Answer from the drawing. Dimensions are ordinates in mm from the lowest x, y and z of the part. A direction names the side the tool comes from. Coordinates: 2 decimals unless noted, no trailing zeros. Write each loop counter-clockwise with the first axis right and the second up, starting at its lowest first coordinate (ties: lowest second). Pieces come first, ordered by that corner, then holes. Notation, with made-up numbers: (-40, -30.5) - (-16, -30.5) arc R20 cw to (-16, 5.5) - close; hole circle Ø3 at (-31, 25.5). An arc over 180 degrees is marked (long way). Return JSON: item names as keys, results as strings.
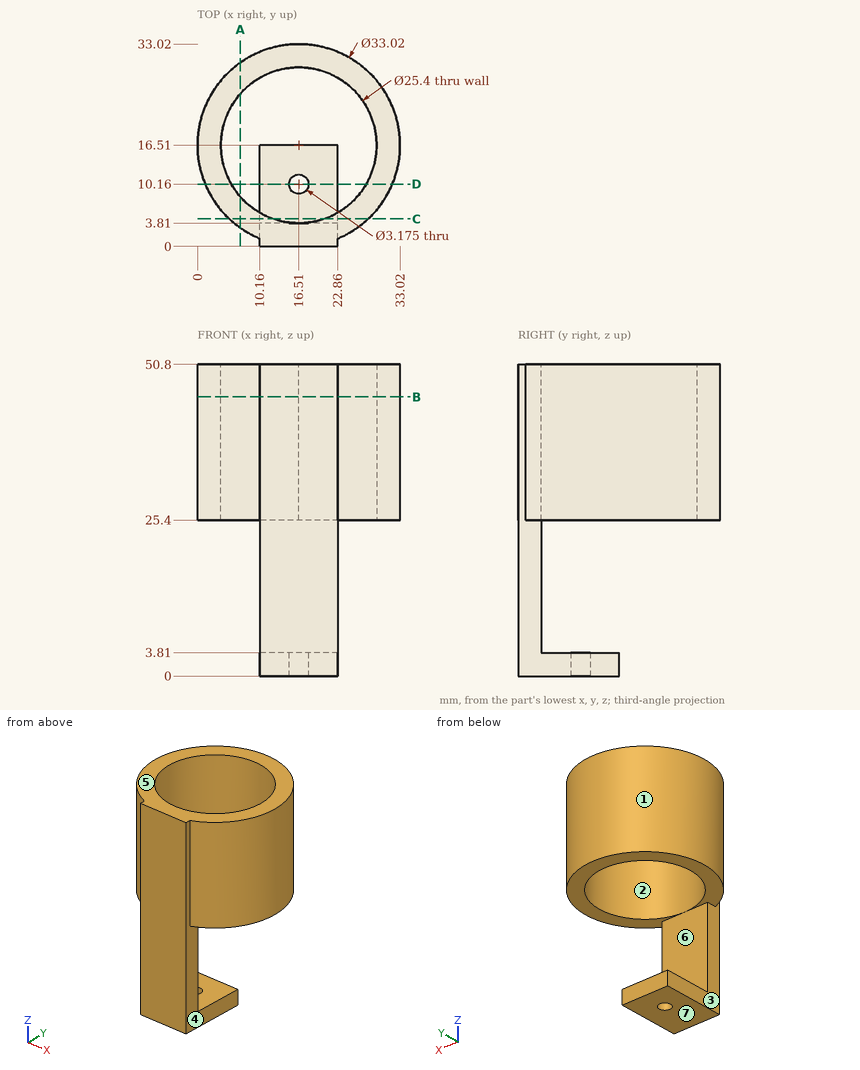
(1) Which of the six approach directions +Z, -Z, +X, -X, +Y, -Y give full straight-line access (tool end or side, diameter ignored) to the marked faces 1, 2 and 3?
Answer:
{"face 1": "+Z, -Z", "face 2": "+Z", "face 3": "-Z, -X, -Y"}
(2) A cutting plane is placed at C-C (y = 4.5). Determine the outline of the cut face in (x, z), and give its area (3 significant figures).
Answer:
{"outline": "(5.18, 25.4) - (12.38, 25.4) - (12.38, 50.8) - (5.18, 50.8) - close; (10.16, 0) - (22.86, 0) - (22.86, 3.81) - (10.16, 3.81) - close; (20.64, 25.4) - (27.84, 25.4) - (27.84, 50.8) - (20.64, 50.8) - close", "area": "414 mm²"}
(3) A cutting plane is placed at D-D (y = 10.16). Determine the outline of the cut face in (x, z).
Answer:
{"outline": "(1.27, 25.4) - (5.51, 25.4) - (5.51, 50.8) - (1.27, 50.8) - close; (10.16, 0) - (14.92, 0) - (14.92, 3.81) - (10.16, 3.81) - close; (18.1, 0) - (22.86, 0) - (22.86, 3.81) - (18.1, 3.81) - close; (27.51, 25.4) - (31.75, 25.4) - (31.75, 50.8) - (27.51, 50.8) - close"}
(4) Flat-ended cylindrical pins translate along their axes: P1, Ø8, axis at y = 8.5, z = 39.5, coming from the -X side; P2, Ø1.9, axis at x = 18.5, z = 1.5, coming from the +Y side; P3, Ø9.5, axis at x = 12.5, y = 24.5, coming from the -Z side. Find the tip coordinate at first contact, or state that the pin passes through.
Answer:
{"P1": "x = 0.49", "P2": "y = 16.51", "P3": "z = 25.4"}
(5) A cutting plane is placed at A-A (x = 7). Determine the outline of the cut face in (y, z), and give its area (3 significant figures).
Answer:
{"outline": "(3.01, 25.4) - (8.09, 25.4) - (8.09, 50.8) - (3.01, 50.8) - close; (24.93, 25.4) - (30.01, 25.4) - (30.01, 50.8) - (24.93, 50.8) - close", "area": "258 mm²"}
(6) Straight lines are drawn through the part: line 1 (X direction, y = 16, z = 42); line 2 (X direction, y = 10, z = 1); line 3 (Z direction, x = 22, y = 28). For each, find the intervals that lie inside material, in ascending order. Write a range as from..to.
Answer:
{"line 1": "0.01..3.82, 29.2..33.01", "line 2": "10.16..14.93, 18.09..22.86", "line 3": "25.4..50.8"}
(7) A cutting plane is placed at B-B (z = 45.5). Determine the outline of the cut face in (x, y).
Answer:
{"outline": "(10.16, 0) - (22.86, 0) - (22.86, 1.27) arc R16.51 ccw (long way) to (10.16, 1.27) - close; hole circle Ø25.4 at (16.51, 16.51)"}
(8) Determine the mould class of the marked faces 4, 5, 6 and 7 for opening direction Z: +Z half, -Z half, draft (parallel to the pull), parting line (faces both ways), or undercut.
Answer:
{"face 4": "draft", "face 5": "+Z half", "face 6": "undercut", "face 7": "-Z half"}
